Design review of the part built by this model. Coordinates are the model's own, in mm. A direction names the side the tool comes from. Coordinates: 2 decimals unless noted, no trailing zeros. Loops run counter-clockwise (first coordinate to the right, second up) from the corner with the lowest first, then second, coordinate; pieces in that order, holes last. Notation, with made-up numbers: (-36.75, 82.5) -> (19.25, 82.5) arc R21 ccw to (19.25, 101.5) -> close; hole circle Ø9 at (31, 57.5). An arc over 180 degrees is marked (long way). One line per item, written item: value. Start each with the question number.
1. Add section B-B on x = 7.5. Write out the cut boundary in (y, z), plus the area to 3 significant figures.
2. Insertion check: pin 1 (3 mm diameter, centred on x = -3, y = -19.5, fed in from +Z); pin 2 (5 mm diameter, centred on x = 24, y = -35.5, fed in from +Z); pin 3 (1.5 mm diameter, centred on x = 32, y = 27.5, fed in from +Z). Each pin has a flat end and moves straight along its axis. Give the tip position at first contact, or say it passes through.
3. Machinability: for faces 1 (the flat face through (25, 49.5, 76)), 2 (the flat face through (25, -2, 15.5)), 3 (the flat face through (-2, -27, 10)), which of the approach directions +Z, -Z, +X, -X, +Y, -Y give a long, thin tool a straight path to every point of the face, cutting with its end or side? Answer none if there is none.
4. Add section D-D on z = 13. Write out the cut boundary in (x, y).
5. Add section C-C on y = -14. Write out the cut boundary in (x, z).
6. For probe 1 along Y at (x, z) = (4, 76); probe 2 along X at (y, z) = (49, 35); probe 3 along Z at (x, y) = (24, -5.5), list the stretches that pass through material, from the lowest coordinate up.
7. Add section A-A on z = 86. Write out the cut boundary in (x, y).
8. Draft analysis for pull direction X (two halves, no side actions). For faces 4 (the flat face through (55, 24, 61)), 5 (the flat face through (25, -24, 0)), 6 (the flat face through (25, 1, -4)), state which applies: pulls with the +X half, pulls with the -X half, needs draft (parallel to the pull), parting line crosses it, or undercut.
```python
from build123d import *

# Parameters (mm, degrees)
F0_W     = 4
F0_H     = 6.48995
F0_W_2   = 49.5
F0_H_2   = 4
F1_DEPTH = 4
F2_DEPTH = 55
F3_DEPTH = 51


with BuildPart() as f1:
    # F0 (on Right) → F1 (new body)
    with BuildSketch(Plane.YZ):
        Polygon((46.5, 0), (0, 0), (-46.5, 0), (-46.5, 3.51005), (-50.5, 3.51005), (-50.5, -4), (0, -4), (46.5, -4), (53.5, -4), (53.5, 124), (49.5, 124), (49.5, 120), (49.5, 29.608211), (49.5, 0), align=None)
        with BuildLine():
            ThreePointArc((31.99437, 10), (16.760368, 2.558245), (0, 0))
            Line((0, 0), (46.5, 0))
            Line((46.5, 0), (49.5, 0))
            Line((49.5, 0), (49.5, 29.608211))
            ThreePointArc((49.5, 29.608211), (41.910065, 18.76592), (31.99437, 10))
        make_face()
        with BuildLine():
            Line((0, 10), (0, 0))
            ThreePointArc((0, 0), (16.760368, 2.558245), (31.99437, 10))
            Line((31.99437, 10), (0, 10))
        make_face()
        Polygon((-46.5, 0), (0, 0), (0, 10), (-4, 10), (-46.5, 10), (-46.5, 3.51005), align=None)
        with BuildLine():
            Line((0, 10), (31.99437, 10))
            ThreePointArc((31.99437, 10), (41.910065, 18.76592), (49.5, 29.608211))
            Line((49.5, 29.608211), (49.5, 120))
            Line((49.5, 120), (0, 120))
            Line((0, 120), (0, 56.181986))
            Line((0, 56.181986), (0, 15.5))
            Line((0, 15.5), (-4, 15.5))
            Line((-4, 15.5), (-4, 10))
            Line((-4, 10), (0, 10))
        make_face()
        with Locations((-48.5, 6.755025)):
            Rectangle(F0_W, F0_H)
        Polygon((-4, 124), (-4, 15.5), (0, 15.5), (0, 56.181986), (0, 120), (0, 124), align=None)
        with Locations((24.75, 122)):
            Rectangle(F0_W_2, F0_H_2)
    extrude(amount=-F1_DEPTH)

    # F0 (on Right) → F2 (join)
    with BuildSketch(Plane.YZ):
        Polygon((46.5, 0), (0, 0), (-46.5, 0), (-46.5, 3.51005), (-50.5, 3.51005), (-50.5, -4), (0, -4), (46.5, -4), (53.5, -4), (53.5, 124), (49.5, 124), (49.5, 120), (49.5, 29.608211), (49.5, 0), align=None)
        with BuildLine():
            ThreePointArc((31.99437, 10), (16.760368, 2.558245), (0, 0))
            Line((0, 0), (46.5, 0))
            Line((46.5, 0), (49.5, 0))
            Line((49.5, 0), (49.5, 29.608211))
            ThreePointArc((49.5, 29.608211), (41.910065, 18.76592), (31.99437, 10))
        make_face()
        with BuildLine():
            Line((0, 10), (31.99437, 10))
            ThreePointArc((31.99437, 10), (41.910065, 18.76592), (49.5, 29.608211))
            Line((49.5, 29.608211), (49.5, 120))
            Line((49.5, 120), (0, 120))
            Line((0, 120), (0, 56.181986))
            Line((0, 56.181986), (0, 15.5))
            Line((0, 15.5), (-4, 15.5))
            Line((-4, 15.5), (-4, 10))
            Line((-4, 10), (0, 10))
        make_face()
        Polygon((-46.5, 0), (0, 0), (0, 10), (-4, 10), (-46.5, 10), (-46.5, 3.51005), align=None)
        with BuildLine():
            Line((0, 10), (0, 0))
            ThreePointArc((0, 0), (16.760368, 2.558245), (31.99437, 10))
            Line((31.99437, 10), (0, 10))
        make_face()
        with Locations((-48.5, 6.755025)):
            Rectangle(F0_W, F0_H)
        Polygon((-4, 124), (-4, 15.5), (0, 15.5), (0, 56.181986), (0, 120), (0, 124), align=None)
        with Locations((24.75, 122)):
            Rectangle(F0_W_2, F0_H_2)
    extrude(amount=F2_DEPTH)

    # F0 (on Right) → F3 (cut)
    with BuildSketch(Plane.YZ):
        with BuildLine():
            Line((0, 10), (31.99437, 10))
            ThreePointArc((31.99437, 10), (41.910065, 18.76592), (49.5, 29.608211))
            Line((49.5, 29.608211), (49.5, 120))
            Line((49.5, 120), (0, 120))
            Line((0, 120), (0, 56.181986))
            Line((0, 56.181986), (0, 15.5))
            Line((0, 15.5), (-4, 15.5))
            Line((-4, 15.5), (-4, 10))
            Line((-4, 10), (0, 10))
        make_face()
        with BuildLine():
            Line((0, 10), (0, 0))
            ThreePointArc((0, 0), (16.760368, 2.558245), (31.99437, 10))
            Line((31.99437, 10), (0, 10))
        make_face()
        Polygon((-46.5, 0), (0, 0), (0, 10), (-4, 10), (-46.5, 10), (-46.5, 3.51005), align=None)
        with Locations((-48.5, 6.755025)):
            Rectangle(F0_W, F0_H)
        with Locations((24.75, 122)):
            Rectangle(F0_W_2, F0_H_2)
    extrude(amount=F3_DEPTH, mode=Mode.SUBTRACT)


solid = f1.part
```
Worked answers:
1. outline: (-50.5, -4) -> (53.5, -4) -> (53.5, 124) -> (49.5, 124) -> (49.5, 29.61) arc R56.18 cw to (31.99, 10) arc R56.18 cw to (0, 0) -> (-46.5, 0) -> (-46.5, 3.51) -> (-50.5, 3.51) -> close; (-4, 15.5) -> (0, 15.5) -> (0, 124) -> (-4, 124) -> close
1. area: 1,780 mm²
2. pin 1: stops at z = 10
2. pin 2: stops at z = 0
2. pin 3: stops at z = 7.62
3. face 1: +Z
3. face 2: -Y
3. face 3: +Z, +X, -X, -Y
4. outline: (-4, -4) -> (0, -4) -> (0, 35.94) -> (51, 35.94) -> (51, -4) -> (55, -4) -> (55, 53.5) -> (-4, 53.5) -> close
5. outline: (-4, -4) -> (55, -4) -> (55, 10) -> (51, 10) -> (51, 0) -> (0, 0) -> (0, 10) -> (-4, 10) -> close
6. probe 1: y = -4 to 0, 49.5 to 53.5
6. probe 2: x = -4 to 0, 51 to 55
6. probe 3: z = -4 to 0
7. outline: (-4, -4) -> (55, -4) -> (55, 53.5) -> (-4, 53.5) -> close; hole (0, 0) -> (51, 0) -> (51, 49.5) -> (0, 49.5) -> close
8. face 4: pulls with the +X half
8. face 5: undercut
8. face 6: needs draft
